from build123d import *

# Parameters (mm, degrees)
F1_DEPTH = 20
F2_W     = 26
F2_H     = 113.192833
F3_DEPTH = 7
F4_R     = 2.75
F5_DEPTH = 170


with BuildPart() as f1:
    # F0 (on Top) → F1 (new body)
    with BuildSketch(Plane.XY):
        Polygon((-34.973299, 75.256209), (-34.973299, -24.743791), (-19.973299, -24.743791), (0.026701, -4.743791), (100.026701, -4.743791), (120.026701, -24.743791), (135.026701, -24.743791), (135.026701, 75.256209), align=None)
    extrude(amount=F1_DEPTH)

    # F2 (on face) → F3 (cut)
    with BuildSketch(Plane.XY.offset(20)):
        with Locations((-19.823299, 26.061079)):
            Rectangle(F2_W, F2_H)
        with Locations((8.116701, 26.061079)):
            Rectangle(F2_W, F2_H)
        with Locations((36.056701, 26.061079)):
            Rectangle(F2_W, F2_H)
        with Locations((63.996701, 26.061079)):
            Rectangle(F2_W, F2_H)
        with Locations((91.936701, 26.061079)):
            Rectangle(F2_W, F2_H)
        with Locations((119.876701, 26.061079)):
            Rectangle(F2_W, F2_H)
    extrude(amount=-F3_DEPTH, mode=Mode.SUBTRACT)

    # F4 (on face) → F5 (cut, through all)
    with BuildSketch(Plane(origin=(-34.973299, 0, 0), x_dir=(0, -1, 0), z_dir=(-1, 0, 0))):
        with Locations((14.743791, 7)):
            Circle(F4_R)
    extrude(amount=-F5_DEPTH, mode=Mode.SUBTRACT)


solid = f1.part
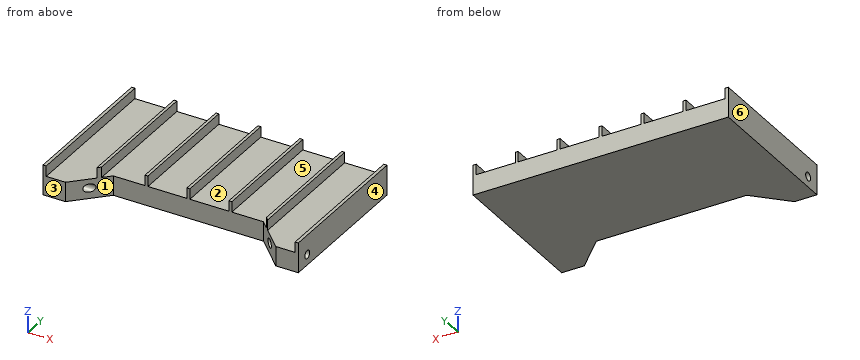
Geometry: final body of the model. Coordinates: model frame, mm. Face numbers are marked on the shaded views. A direction names the side the tool comes from. Give positions to 0.01 mm unless a question says otherwise; leave off trailing zeros. Write each loop counter-clockwise with the first axis right and the second up, starting at its lowest first coordinate (ties: lowest second). Pieces come first, ordered by that corner, then holes. Notation, with made-up numbers: M 41,-38 L 70,-38 A13 cw 70,-20 Z; hole C 56.25,34.5 d4. An arc over 180 degrees is marked long. Answer in a Markdown table with one row per item. Add a question column.
(1) Section D-D on x = 34. Return loops of the section in (y, z), and give its area (3 significant figures).
(2) Section B-B on z = 2. Return loops of the section in (x, y).
(3) Reachability of the marked faces 1, 2 and 3 from +Z, -Z, +X, -X, +Y, -Y: full face, straight path, thin tool, end or side. Return the list, or none.
(4) Mould query, pull axis X, two halves, no side actions, for the marked faces 4, 5 and 6. Classes: +X half, -X half, draft (parallel to the pull), parting line (faces both ways), or undercut.
(5) Section A-A on z = 16. Return loops of the section in (x, y).
(6) First-contact query: pin 1 (4 mm diameter, centred on x = -0.5, z = 12, fed in from -Y); pin 2 (10 mm diameter, centred on x = 0.5, y = 13.5, fed in from +Z). Flat tips, straight axial feed; report the tip coordinate or a pass-through.
(7) Section C-C on y = 3. Return loops of the section in (x, z), and give its area (3 significant figures).
(8) Ray query, line 1 (X direction, y = -9, z = 14.5); line 2 (Y direction, x = 126.75, z = 7); line 3 (Y direction, x = -11, z = 6.75). Return the intervals inside material, ascending.
Result set:
| question | item | result |
|---|---|---|
| 1 | outline | M -4.74,0 L 75.26,0 L 75.26,13 L -4.74,13 Z |
| 1 | area | 1,040 mm^2 |
| 2 | outline | M -34.97,-24.74 L -19.97,-24.74 L 0.03,-4.74 L 100.03,-4.74 L 120.03,-24.74 L 135.03,-24.74 L 135.03,75.26 L -34.97,75.26 Z |
| 3 | face 1 | +Z, -Z, -Y |
| 3 | face 2 | +Z, +Y, -Y |
| 3 | face 3 | +Z, -Z, +X, -X, -Y |
| 4 | face 4 | +X half |
| 4 | face 5 | undercut |
| 4 | face 6 | -X half |
| 5 | outline | M -34.97,-24.74 L -32.82,-24.74 L -32.82,75.26 L -34.97,75.26 Z; M -6.82,-11.59 L -4.88,-9.65 L -4.88,75.26 L -6.82,75.26 Z; M 21.12,-4.74 L 23.06,-4.74 L 23.06,75.26 L 21.12,75.26 Z; M 49.06,-4.74 L 51,-4.74 L 51,75.26 L 49.06,75.26 Z; M 77,-4.74 L 78.94,-4.74 L 78.94,75.26 L 77,75.26 Z; M 104.94,-9.65 L 106.88,-11.59 L 106.88,75.26 L 104.94,75.26 Z; M 132.88,-24.74 L 135.03,-24.74 L 135.03,75.26 L 132.88,75.26 Z |
| 6 | pin 1 | stops at y = -7.27 |
| 6 | pin 2 | stops at z = 13 |
| 7 | outline | M -34.97,0 L 135.03,0 L 135.03,20 L 132.88,20 L 132.88,13 L 106.88,13 L 106.88,20 L 104.94,20 L 104.94,13 L 78.94,13 L 78.94,20 L 77,20 L 77,13 L 51,13 L 51,20 L 49.06,20 L 49.06,13 L 23.06,13 L 23.06,20 L 21.12,20 L 21.12,13 L -4.88,13 L -4.88,20 L -6.82,20 L -6.82,13 L -32.82,13 L -32.82,20 L -34.97,20 Z |
| 7 | area | 2,310 mm^2 |
| 8 | line 1 | x = -34.97 to -32.82, -6.82 to -4.88, 104.94 to 106.88, 132.88 to 135.03 |
| 8 | line 2 | y = -24.74 to -17.49, -11.99 to 75.26 |
| 8 | line 3 | y = -12.01 to 75.26 |
